from build123d import *

# Parameters (mm, degrees)
SKETCH1_R           = 138.90625
BOSS_EXTRUDE1_DEPTH = 1.905
SKETCH2_R           = 27.94
BOSS_EXTRUDE2_DEPTH = 1.905
SKETCH3_R           = 2.0828
CUT_EXTRUDE1_DEPTH  = 1.524
FILLET1_R           = 5.08
SKETCH4_W           = 1.524
SKETCH4_H           = 6.35
CUT_EXTRUDE2_DEPTH  = 1.524
CIRPATTERN1_COUNT   = 8
CUT_EXTRUDE3_DEPTH  = 197.452339266


with BuildPart() as part:
    # Sketch1 → Boss-Extrude1 (new body)
    with BuildSketch(Plane(origin=(0, 0, 0), x_dir=(1, 0, 0), z_dir=(0, 1, 0))):
        with Locations(Location((0, 0, 0), (0, 0, 90))):
            Circle(SKETCH1_R)
        with BuildLine():
            ThreePointArc((-97.038504037, 90.303311946), (-122.466006281, 50.727080731), (-132.470668481, 4.7625))
            Line((-132.470668481, 4.7625), (-11.497692091, 4.7625))
            Line((-11.497692091, 4.7625), (-97.038504037, 90.303311946))
        make_face(mode=Mode.SUBTRACT)
        with BuildLine():
            ThreePointArc((-132.470668481, -4.7625), (-122.466006281, -50.727080731), (-97.038504037, -90.303311946))
            Line((-97.038504037, -90.303311946), (-11.497692091, -4.7625))
            Line((-11.497692091, -4.7625), (-132.470668481, -4.7625))
        make_face(mode=Mode.SUBTRACT)
        with BuildLine():
            ThreePointArc((-90.303311946, -97.038504037), (-50.727080731, -122.466006281), (-4.7625, -132.470668481))
            Line((-4.7625, -132.470668481), (-4.7625, -11.497692091))
            Line((-4.7625, -11.497692091), (-90.303311946, -97.038504037))
        make_face(mode=Mode.SUBTRACT)
        with BuildLine():
            ThreePointArc((4.7625, -132.470668481), (50.727080731, -122.466006281), (90.303311946, -97.038504037))
            Line((90.303311946, -97.038504037), (4.7625, -11.497692091))
            Line((4.7625, -11.497692091), (4.7625, -132.470668481))
        make_face(mode=Mode.SUBTRACT)
        with BuildLine():
            ThreePointArc((97.038504037, -90.303311946), (122.466006281, -50.727080731), (132.470668481, -4.7625))
            Line((132.470668481, -4.7625), (11.497692091, -4.7625))
            Line((11.497692091, -4.7625), (97.038504037, -90.303311946))
        make_face(mode=Mode.SUBTRACT)
        with BuildLine():
            ThreePointArc((132.470668481, 4.7625), (122.466006281, 50.727080731), (97.038504037, 90.303311946))
            Line((97.038504037, 90.303311946), (11.497692091, 4.7625))
            Line((11.497692091, 4.7625), (132.470668481, 4.7625))
        make_face(mode=Mode.SUBTRACT)
        with BuildLine():
            ThreePointArc((90.303311946, 97.038504037), (50.727080731, 122.466006281), (4.7625, 132.470668481))
            Line((4.7625, 132.470668481), (4.7625, 11.497692091))
            Line((4.7625, 11.497692091), (90.303311946, 97.038504037))
        make_face(mode=Mode.SUBTRACT)
        with BuildLine():
            ThreePointArc((-4.7625, 132.470668481), (-50.612212833, 122.513523034), (-90.121152576, 97.207701714))
            Line((-90.121152576, 97.207701714), (-4.7625, 11.497692091))
            Line((-4.7625, 11.497692091), (-4.7625, 132.470668481))
        make_face(mode=Mode.SUBTRACT)
    extrude(amount=BOSS_EXTRUDE1_DEPTH)

    # Sketch2 → Boss-Extrude2 (add)
    with BuildSketch(Plane(origin=(0, 1.905, 0), x_dir=(1, 0, 0), z_dir=(0, 1, 0))):
        Circle(SKETCH2_R)
    extrude(amount=-BOSS_EXTRUDE2_DEPTH)

    # Sketch3 → Cut-Extrude1 (cut)
    with BuildSketch(Plane(origin=(0, 1.905, 0), x_dir=(1, 0, 0), z_dir=(0, 1, 0))):
        with Locations(Location((0, 23.8125, 0), (0, 0, 270))):
            Circle(SKETCH3_R)
        with Locations(Location((20.622229928, 11.90625, 0), (0, 0, 270))):
            Circle(SKETCH3_R)
        with Locations(Location((20.622229928, -11.90625, 0), (0, 0, 270))):
            Circle(SKETCH3_R)
        with Locations(Location((0, -23.8125, 0), (0, 0, 270))):
            Circle(SKETCH3_R)
        with Locations(Location((-20.622229928, -11.90625, 0), (0, 0, 270))):
            Circle(SKETCH3_R)
        with Locations(Location((-20.622229928, 11.90625, 0), (0, 0, 270))):
            Circle(SKETCH3_R)
    extrude(amount=-CUT_EXTRUDE1_DEPTH, mode=Mode.SUBTRACT)

    # Fillet1
    fillet1_edges = [part.edges().sort_by_distance(p)[0] for p in [
        (-16.072522378, 0.9525, -22.854269282),
        (4.7625, 0.9525, -27.531113195),
        (22.835032879, 0.9525, -16.099840788),
        (27.531113195, 0.9525, 4.7625),
        (16.099840788, 0.9525, 22.835032879),
        (-4.7625, 0.9525, 27.531113195),
        (-22.835032879, 0.9525, 16.099840788),
        (-27.531113195, 0.9525, -4.7625),
        (-22.835032879, 0.9525, -16.099840788),
        (-4.7625, 0.9525, -27.531113195),
        (16.099840788, 0.9525, -22.835032879),
        (27.531113195, 0.9525, -4.7625),
        (22.835032879, 0.9525, 16.099840788),
        (4.7625, 0.9525, 27.531113195),
        (-16.099840788, 0.9525, 22.835032879),
        (-27.531113195, 0.9525, 4.7625),
    ]]
    fillet(fillet1_edges, radius=FILLET1_R)

    # Sketch4 → Cut-Extrude2 (cut)
    with BuildSketch(Plane(origin=(0, 1.905, 0), x_dir=(1, 0, 0), z_dir=(0, 1, 0))):
        with Locations((0, 135.73125)):
            Rectangle(SKETCH4_W, SKETCH4_H)
    cut_extrude2 = extrude(amount=-CUT_EXTRUDE2_DEPTH, mode=Mode.SUBTRACT)

    # CirPattern1: Cut-Extrude2 ×8 about axis
    cirpattern1_axis = Axis((0, 0, 0), (0, 1, 0))
    for i in range(1, CIRPATTERN1_COUNT):
        add(cut_extrude2.rotate(cirpattern1_axis, i * 360 / CIRPATTERN1_COUNT), mode=Mode.SUBTRACT)

    # Sketch5 → Cut-Extrude3 (cut, through all)
    with BuildSketch(Plane(origin=(0, 1.905, 0), x_dir=(1, 0, 0), z_dir=(0, 1, 0))):
        Polygon((3.666174209, 6.35), (-3.666174209, 6.35), (-7.332348419, 0), (-3.666174209, -6.35), (3.666174209, -6.35), (7.332348419, 0), align=None)
    extrude(amount=-CUT_EXTRUDE3_DEPTH, mode=Mode.SUBTRACT)


solid = part.part
Read the model definition and answer for the solid it produces. Units are mm, in the model's axes. A direction names the side the tool comes from. Coordinates: 2 decimals unless noted, no trailing zeros. Loops run counter-clockwise (first coordinate to the right, second up) from the corner with the lowest first, then second, coordinate; pieces in that order, holes last. Notation, with made-up numbers: (31.5, -26.5) -> (61.5, -26.5) arc R22 ccw to (61.5, -14.5) -> close; hole circle Ø4 at (44.25, 76.5). An arc over 180 degrees is marked (long way). Answer in a Markdown table with one row per item.
Item 1: A cutting plane is placed at A-A on x = 113. Determine the outline of the cut face in (y, z) (1 decimal).
Returned:
| item | result |
|---|---|
| outline | (0, -80.8) -> (1.9, -80.8) -> (1.9, -69.3) -> (0, -69.3) -> close; (0, -4.8) -> (1.9, -4.8) -> (1.9, 4.8) -> (0, 4.8) -> close; (0, 69.3) -> (1.9, 69.3) -> (1.9, 80.8) -> (0, 80.8) -> close |
Item 2: For faces 1 (the flat face through (-2, 0, -29)), 2 (the cylindrical face through (-51.34, 0.94, 122.21)), determine the directions among +Z, -Z, +X, -X, +Y, -Y from which every point of the face is accessible in a straight line to the end or side of a thin tool.
Returned:
| item | result |
|---|---|
| face 1 | +Z, -Z, +X, -X, -Y |
| face 2 | +Y, -Y |
Item 3: Straight lines are drawn through the part: line 1 along X through (y, z) = (1.7, -80.5); line 2 along X through (y, z) = (1.7, 23); line 3 along X through (y, z) = (1, -41). For each, find the intervals that lie inside material, in ascending order. Write a range as [from, to].
Returned:
| item | result |
|---|---|
| line 1 | x = [-113.2, -105.31], [-87.24, -73.48], [-4.76, 4.76], [73.76, 87.24], [105.31, 113.2] |
| line 2 | x = [-136.99, -130.55], [-29.74, -1.92], [1.92, 29.74], [130.55, 136.99] |
| line 3 | x = [-132.72, -126.06], [-47.74, -34.14], [-4.76, 4.76], [34.26, 47.74], [126.06, 132.72] |
Item 4: For a pull along X with two mould halves and no side action, classify faces 3 (the flat face through (29, 1.905, 2)), 4 (the cylindrical face through (122.72, 0.94, -50.11)), 5 (the cylindrical face through (123.23, 0.94, -64.1)), 6 (the flat face through (-60.847, 0.939, -54.112)) as released by +X, released by -X, zero draft, split by the parting line, or undercut.
Returned:
| item | result |
|---|---|
| face 3 | zero draft |
| face 4 | undercut |
| face 5 | split by the parting line |
| face 6 | undercut |
Item 5: A cutting plane is placed at B-B on x = -35. Determine the outline of the cut face in (y, z) (1 decimal), plus the area to 3 significant figures.
Returned:
| item | result |
|---|---|
| outline | (0, -134.4) -> (1.9, -134.4) -> (1.9, -127.9) -> (0, -127.9) -> close; (0, -41.9) -> (1.9, -41.9) -> (1.9, -28.3) -> (0, -28.3) -> close; (0, -4.8) -> (1.9, -4.8) -> (1.9, 4.8) -> (0, 4.8) -> close; (0, 28.3) -> (1.9, 28.3) -> (1.9, 41.7) -> (0, 41.7) -> close; (0, 127.9) -> (1.9, 127.9) -> (1.9, 134.4) -> (0, 134.4) -> close |
| area | 94.7 mm^2 |
Item 6: A cutting plane is placed at C-C on y = 1.45. Give the number of separate pieces and of enclosed holes in the cut face, plus the area to 3 significant figures.
Returned:
| item | result |
|---|---|
| separate pieces | 1 |
| enclosed holes | 15 |
| area | 15,600 mm^2 |
Item 7: Each of these flat-tipped pins is pushed along its axis until it touches: P1, Ø12, axis at x = 98.5, z = -108.5, coming from the +Y side; P2, Ø1, axis at y = 1, z = 77, coming from the -X side; P3, Ø0.5, axis at x = 0, z = -137.5, coming from the +Y side; P4, Ø1, axis at x = -70.5, y = 0.5, coming from the -Z side. Where does it stop, or does it pass through?
Returned:
| item | result |
|---|---|
| P1 | passes through |
| P2 | stops at x = -115.94 |
| P3 | stops at y = 0.38 |
| P4 | stops at z = -119.98 |
